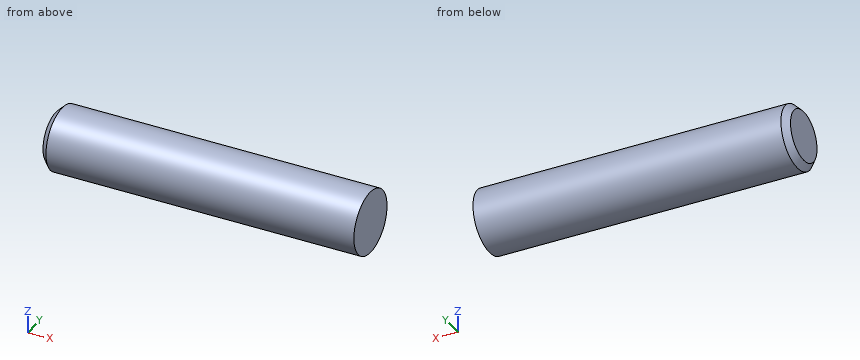
from build123d import *

# Parameters (mm, degrees)
EXTRUDE1_DEPTH        = 7.9375
EXTRUDE1_DEPTH_BACK   = 7.9375
SKETCH2_R             = 1.5875
CHAMFER1_SIZE         = 0.3175
DELETEFACE1_START     = 7.6199999
DELETEFACE1_OUTLINE_R = 1.5875
DELETEFACE1_DEPTH     = 0.3175001


# Read off the part's stored shape, not the designer's step: DeleteFace1
with BuildPart() as part:
    # Sketch2 → Extrude1 (new, two sides: drawn at the far end of the back side and taken through both)
    with BuildSketch(Plane(origin=(0, 0, 0), x_dir=(0, 0, -1), z_dir=(1, 0, 0)).offset(-EXTRUDE1_DEPTH_BACK)):
        Circle(SKETCH2_R)
    extrude(amount=EXTRUDE1_DEPTH + EXTRUDE1_DEPTH_BACK)

    # Chamfer1
    chamfer1_edges = [part.edges().sort_by_distance(p)[0] for p in [
        (-7.9375, 0, 1.5875),
        (7.9375, 0, 1.5875),
    ]]
    chamfer(chamfer1_edges, length=CHAMFER1_SIZE)

    # DeleteFace1 outline → DeleteFace1 (add)
    with BuildSketch(Plane.YZ.offset(DELETEFACE1_START)):
        Circle(DELETEFACE1_OUTLINE_R)
    extrude(amount=DELETEFACE1_DEPTH)


solid = part.part
Input: part model. Units: mm. Frame: model coordinates. Give positions to 0.01 mm unless a question says otherwise; leave off trailing zeros. Write each loop counter-clockwise with the first axis right and the second up, starting at its lowest first coordinate (ties: lowest second). Pieces come first, ordered by that corner, then holes. Notation, with made-up numbers: M -16,-37.5 L -7,-37.5 A21 ccw -7,-9.5 Z; hole C 23,29.5 d2. An arc over 180 degrees is marked long. Write item = value, one per line. Start each with the question number.
1) Cut plane A-A on x = -2.25. Return the cut outline in (y, z) (1 decimal).
2) First-contact query: pin 1 Ø1.5 at (x, y) = (-6, 1) entering from +Z. Flat tip, straight axial feed; report the tip coordinate or a pass-through.
3) Material intervals for line 1 along Y through (x, z) = (7, 0.95); line 2 along Z through (x, y) = (-2.5, 0.25), sorted ascending. Write a range as [from, to].
Solved:
q1.outline = C 0,0 d3.2
q2.pin_1 = 1.57
q3.line_1 = [-1.27, 1.27]
q3.line_2 = [-1.57, 1.57]
